```python
from build123d import *

# Parameters (mm, degrees)
F0_W      = 139.7
F0_H      = 76.2
F1_DEPTH  = 25.4
F2_SIZE   = 5.08
F3_W      = 144.291125
F3_H      = 81.529271
F4_DEPTH  = 2.54
F1_FACE_W = 137.16
F1_FACE_H = 25.4
F5_DEPTH  = 12.7
F6_W      = 7.62
F6_H      = 7.62
F7_DEPTH  = 12.7
F8_SIZE   = 2.54
F9_SIZE   = 2.54
F10_SIZE  = 2.54
F11_SIZE  = 2.54


with BuildPart() as f1:
    # F0 (on Top) → F1 (new body)
    with BuildSketch(Plane.XY):
        with BuildLine():
            ThreePointArc((76.2, 36.83), (73.968154, 42.218154), (68.58, 44.45))
            Line((68.58, 44.45), (-68.58, 44.45))
            ThreePointArc((-68.58, 44.45), (-73.968154, 42.218154), (-76.2, 36.83))
            Line((-76.2, 36.83), (-76.2, -36.83))
            ThreePointArc((-76.2, -36.83), (-73.968154, -42.218154), (-68.58, -44.45))
            Line((-68.58, -44.45), (68.58, -44.45))
            ThreePointArc((68.58, -44.45), (73.968154, -42.218154), (76.2, -36.83))
            Line((76.2, -36.83), (76.2, 36.83))
        make_face()
        Rectangle(F0_W, F0_H, mode=Mode.SUBTRACT)
    extrude(amount=F1_DEPTH)

    # F2
    f2_edges = [f1.edges().sort_by_distance(p)[0] for p in [
        (-69.85, 38.1, 12.7),
        (-69.85, -38.1, 12.7),
        (69.85, 38.1, 12.7),
        (69.85, -38.1, 12.7),
    ]]
    chamfer(f2_edges, length=F2_SIZE)

    # F3 (on Top) → F4 (join)
    with BuildSketch(Plane.XY):
        with Locations((-0.039962, 0.51033)):
            Rectangle(F3_W, F3_H)
    extrude(amount=F4_DEPTH)

    # F1_face (on face) → F5 (join)
    with BuildSketch(Plane(origin=(0, -44.45, 12.7), x_dir=(1, 0, 0), z_dir=(0, -1, 0))):
        Rectangle(F1_FACE_W, F1_FACE_H)
    extrude(amount=F5_DEPTH)

    # F6 (on face) → F7 (join)
    with BuildSketch(Plane.XY.offset(25.4)):
        with Locations((26.67, -48.26)):
            Rectangle(F6_W, F6_H)
        with Locations((-26.67, -48.26)):
            Rectangle(F6_W, F6_H)
    extrude(amount=F7_DEPTH)

    # F8
    f8_edges = [f1.edges().sort_by_distance(p)[0] for p in [
        (30.48, -44.45, 31.75),
    ]]
    chamfer(f8_edges, length=F8_SIZE)

    # F9
    f9_edges = [f1.edges().sort_by_distance(p)[0] for p in [
        (22.86, -44.45, 31.75),
        (22.86, -52.07, 31.75),
    ]]
    chamfer(f9_edges, length=F9_SIZE)

    # F10
    f10_edges = [f1.edges().sort_by_distance(p)[0] for p in [
        (30.48, -52.07, 31.75),
    ]]
    chamfer(f10_edges, length=F10_SIZE)

    # F11
    f11_edges = [f1.edges().sort_by_distance(p)[0] for p in [
        (-30.48, -44.45, 31.75),
        (-22.86, -44.45, 31.75),
        (-30.48, -52.07, 31.75),
        (-22.86, -52.07, 31.75),
    ]]
    chamfer(f11_edges, length=F11_SIZE)


solid = f1.part
```
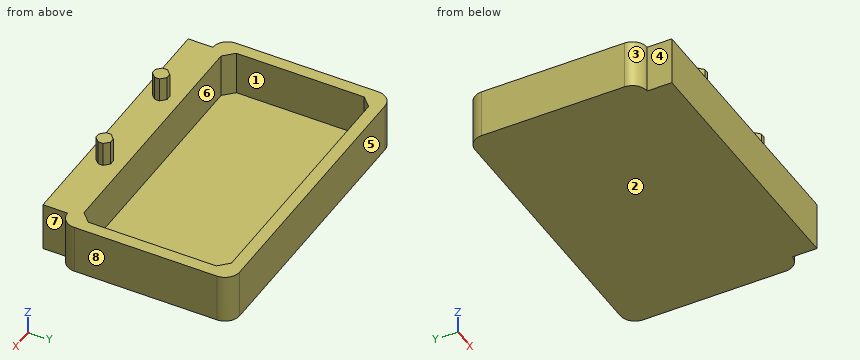
Part model, mm, in its own coordinate system. Face numbers are marked on the shaded views. A direction names the side the tool comes from. Round coordinates to 2 decimals unless told otherwise and drop trailing zeros. Loops run counter-clockwise (first coordinate to the right, second up) from the corner with the lowest first, then second, coordinate; pieces in that order, holes last.
Item 1: Cut at A-A, the plane z = 32.5. Give the cut face in (x, y).
Item 2: Cut at C-C, the plane x = -59. Give the cut face in (y, z).
Item 3: Drop flat-ended pins along their axis: P1, Ø6.5, axis at y = -50, z = 11, coming from the +X side; P2, Ø6.5, axis at y = -50.5, z = 17.5, coming from the -X side; P3, Ø0.8, axis at y = -48.5, z = 30.5, coming from the -X side. Give the stop position or say it passes through.
Item 4: 3-axis set-ups, long thin cutter, end or side, ignore diameter. For the marked faces 4, 5, 6, 7 and 8: which of +Z, -Z, +X, -X, +Y, -Y reach the whole face in a straight line?
Item 5: Drill centre lines: line 1 (Y direction, x = 20, z = 14.5); line 2 (X direction, y = 33, z = 16.5); line 3 (Z direction, x = 10, y = -40). Where is each one in solid material? Low to high.
Item 6: Cut at B-B, the plane z = 7. Give the cut face in (x, y), then the cut area to 3 significant figures.
Item 7: Cut at D-D, the plane y = 12. Give the cut face in (x, z).
Item 8: Mould opens along Y. For the marked faces 1, 2 and 3 say: +Y half, -Y half, draft (parallel to the pull), parting line (faces both ways), or undercut.
A:
1. outline: (-30.48, -49.53) - (-27.94, -52.07) - (-25.4, -52.07) - (-22.86, -49.53) - (-22.86, -46.99) - (-25.4, -44.45) - (-27.94, -44.45) - (-30.48, -46.99) - close; (22.86, -49.53) - (25.4, -52.07) - (27.94, -52.07) - (30.48, -49.53) - (30.48, -46.99) - (27.94, -44.45) - (25.4, -44.45) - (22.86, -46.99) - close
2. outline: (-57.15, 0) - (44.45, 0) - (44.45, 25.4) - (38.1, 25.4) - (38.1, 2.54) - (-38.1, 2.54) - (-38.1, 25.4) - (-57.15, 25.4) - close
3. P1: stops at x = 68.58
3. P2: stops at x = -68.58
3. P3: stops at x = -30.48
4. face 4: +Z, -Z, -X, -Y
4. face 5: +Z, -Z, +X, -X, +Y
4. face 6: +Z
4. face 7: +Z, -Z, +X, -Y
4. face 8: +Z, -Z, +X, +Y, -Y
5. line 1: y = -57.15 to -38.1, 38.1 to 44.45
5. line 2: x = -76.2 to -69.85, 69.85 to 76.2
5. line 3: z = 0 to 25.4
6. outline: (-76.2, -36.83) arc R7.62 ccw to (-68.58, -44.45) - (-68.58, -57.15) - (68.58, -57.15) - (68.58, -44.45) arc R7.62 ccw to (76.2, -36.83) - (76.2, 36.83) arc R7.62 ccw to (68.58, 44.45) - (-68.58, 44.45) arc R7.62 ccw to (-76.2, 36.83) - close; hole (-69.85, -33.02) - (-64.77, -38.1) - (64.77, -38.1) - (69.85, -33.02) - (69.85, 33.02) - (64.77, 38.1) - (-64.77, 38.1) - (-69.85, 33.02) - close
6. area: 4,650 mm2
7. outline: (-76.2, 0) - (76.2, 0) - (76.2, 25.4) - (69.85, 25.4) - (69.85, 2.54) - (-69.85, 2.54) - (-69.85, 25.4) - (-76.2, 25.4) - close
8. face 1: undercut
8. face 2: draft
8. face 3: -Y half
